Input: part model. Units: mm. Frame: model coordinates. A direction names the side the tool comes from. Round coordinates to 2 decimals unless told otherwise and drop trailing zeros. Loops run counter-clockwise (first coordinate to the right, second up) from the corner with the lowest first, then second, coordinate; pieces in that order, holes last.
(1) Line query: line 1 (X direction, y = 16, z = 2.5) (1 decimal); line 2 (Y direction, x = 0, z = 4.75); line 3 (X direction, y = 22.5, z = 8.5). Output: solid intervals per line, ascending.
(2) Cut plane B-B, the plane y = 10. Output: boundary loops of the cut face in (x, z) (3 decimals), and give its area (3 significant figures).
(3) Cut plane A-A, the plane x = 20.5. Output: boundary loops of the cut face in (y, z), and give its area (3 significant figures).
(4) Draft query along X for faces 4 (the face through (45.974, 16, 10)), 5 (the face through (50, 16, 14.224)), 6 (the face through (30, 19.05, 16)). Return one class per face: released by +X, released by -X, zero draft, split by the parting line, or undercut.
(5) Cut plane C-C, the plane z = 4. Output: boundary loops of the cut face in (x, y) (3 decimals), and give its area (3 significant figures).
(6) Cut plane D-D, the plane x = 3. Output: boundary loops of the cut face in (y, z).
(7) Access query for faces 1 (the face through (30, 12.7, 16)), 2 (the face through (51, 4.762, 9)), 3 (the face through (30, 16, 25.4)). Directions: +Z, -Z, +X, -X, +Y, -Y. A direction counts if a zero-diameter tool reaches every point of the face in a straight line with its end or side. Return the directions, or none.
(8) First-contact query: pin 1 Ø8 at (y, z) = (28, 34.5) entering from +X (3 decimals); pin 2 Ø1 at (x, y) = (11.5, 5) entering from -Z; pin 3 Ø1.9 at (x, y) = (36.5, 16.5) entering from +Z; pin 4 Ø10 at (x, y) = (14, 26.5) entering from +Z. Flat tips, straight axial feed; report the tip coordinate or a pass-through.
from build123d import *

# Parameters (mm, degrees)
F1_DEPTH  = 41.275
F3_DEPTH  = 31.751
F5_DEPTH  = 69.851
F6_W      = 22.225
F6_H      = 7.874
F7_DEPTH  = 8.001
F8_R      = 9.525
F9_DEPTH  = 11.176
F10_R     = 1.7272
F11_DEPTH = 31.751
F13_DEPTH = 6.35
F14_R     = 9.525
F15_DEPTH = 12.701
F17_DEPTH = 25.4
F18_R     = 1.7272
F19_DEPTH = 31.751


with BuildPart() as f1:
    # F0 (on Top) → F1 (new body)
    with BuildSketch(Plane.XY):
        with BuildLine():
            ThreePointArc((0, 31.75), (-15.875, 15.875), (0, 0))
            Line((0, 0), (53.975, 0))
            Line((53.975, 0), (53.975, 31.75))
            Line((53.975, 31.75), (0, 31.75))
        make_face()
    extrude(amount=F1_DEPTH)

    # F2 (on face) → F3 (cut, through all)
    with BuildSketch(Plane.XZ):
        Polygon((44.45, 6.35), (44.45, 41.275), (-15.875, 41.275), (-15.875, 12.7), (15.875, 12.7), (15.875, 6.35), align=None)
    extrude(amount=-F3_DEPTH, mode=Mode.SUBTRACT)

    # F4 (on face) → F5 (cut, through all)
    with BuildSketch(Plane.YZ.offset(53.975)):
        with BuildLine():
            ThreePointArc((0, 25.4), (4.6496798487, 36.6253201513), (15.875, 41.275))
            Line((15.875, 41.275), (0, 41.275))
            Line((0, 41.275), (0, 25.4))
        make_face()
        with BuildLine():
            ThreePointArc((15.875, 41.275), (27.1003201513, 36.6253201513), (31.75, 25.4))
            Line((31.75, 25.4), (31.75, 41.275))
            Line((31.75, 41.275), (15.875, 41.275))
        make_face()
    extrude(amount=-F5_DEPTH, mode=Mode.SUBTRACT)

    # F6 (on face) → F7 (cut)
    with BuildSketch(Plane.YZ.offset(53.975)):
        with Locations((15.875, 10.287)):
            Rectangle(F6_W, F6_H)
    extrude(amount=-F7_DEPTH, mode=Mode.SUBTRACT)

    # F8 (on face) → F9 (join)
    with BuildSketch(Plane.YZ.offset(53.975)):
        with Locations((15.875, 25.4)):
            Circle(F8_R)
    extrude(amount=F9_DEPTH)

    # F10 (on face) → F11 (cut, through all)
    with BuildSketch(Plane.XZ):
        with Locations((49.2125, 10.287)):
            Circle(F10_R)
    extrude(amount=-F11_DEPTH, mode=Mode.SUBTRACT)

    # F12 (on face) → F13 (cut)
    with BuildSketch(Plane.XY.offset(12.7)):
        with BuildLine():
            ThreePointArc((0, 31.75), (11.2253201513, 27.1003201513), (15.875, 15.875))
            Line((15.875, 15.875), (15.875, 31.75))
            Line((15.875, 31.75), (0, 31.75))
        make_face()
        with BuildLine():
            Line((15.875, 0), (15.875, 15.875))
            ThreePointArc((15.875, 15.875), (11.2253201513, 4.6496798487), (0, 0))
            Line((0, 0), (15.875, 0))
        make_face()
    extrude(amount=-F13_DEPTH, mode=Mode.SUBTRACT)

    # F14 (on face) → F15 (cut, through all)
    with BuildSketch(Plane.XY.offset(12.7)):
        with Locations((0, 15.875)):
            Circle(F14_R)
    extrude(amount=-F15_DEPTH, mode=Mode.SUBTRACT)

    # F16 (on Top) → F17 (join)
    with BuildSketch(Plane.XY):
        with BuildLine():
            Line((44.45, 19.05), (15.5542598667, 19.05))
            ThreePointArc((15.5542598667, 19.05), (15.875, 15.875), (15.5542598667, 12.7))
            Line((15.5542598667, 12.7), (44.45, 12.7))
            Line((44.45, 12.7), (44.45, 19.05))
        make_face()
    extrude(amount=F17_DEPTH)

    # F18 (on face) → F19 (cut, through all)
    with BuildSketch(Plane(origin=(0, 31.75, 0), x_dir=(-1, 0, 0), z_dir=(0, 1, 0))):
        with Locations((4.8054051585, 7.3282429948)):
            Circle(F18_R)
    extrude(amount=-F19_DEPTH, mode=Mode.SUBTRACT)


solid = f1.part
Reported:
1. line 1: x = -15.9 to -9.5, 9.5 to 54
1. line 2: y = 0 to 6.35, 25.4 to 31.75
1. line 3: x = -14.43 to -6.84, 6.84 to 14.43, 44.45 to 45.97
2. outline: (-14.748, 0) - (-7.497, 0) - (-7.497, 12.7) - (-14.748, 12.7) - close; (7.497, 0) - (53.975, 0) - (53.975, 6.35) - (45.974, 6.35) - (45.974, 14.224) - (53.975, 14.224) - (53.975, 17.903) - (65.151, 17.903) - (65.151, 32.897) - (53.975, 32.897) - (53.975, 40.148) - (44.45, 40.148) - (44.45, 6.35) - (14.748, 6.35) - (14.748, 12.7) - (7.497, 12.7) - close
2. area: 860 mm2
3. outline: (0, 0) - (31.75, 0) - (31.75, 6.35) - (19.05, 6.35) - (19.05, 25.4) - (12.7, 25.4) - (12.7, 6.35) - (0, 6.35) - close
3. area: 323 mm2
4. face 4: released by +X
4. face 5: zero draft
4. face 6: undercut
5. outline: (0, 0) - (53.975, 0) - (53.975, 31.75) - (0, 31.75) arc R15.875 ccw to start; hole circle Ø19.05 at (0, 15.875)
5. area: 1,820 mm2
6. outline: (0, 0) - (6.83, 0) - (6.83, 12.7) - (0.29, 12.7) - (0.29, 6.35) - (0, 6.35) - close; (24.92, 0) - (31.75, 0) - (31.75, 6.35) - (31.46, 6.35) - (31.46, 12.7) - (24.92, 12.7) - close
7. face 1: +Z, -Y
7. face 2: +X
7. face 3: +Z, -X, +Y, -Y
8. pin 1: stops at x = 53.975
8. pin 2: stops at z = 0
8. pin 3: stops at z = 25.4
8. pin 4: stops at z = 12.7
